Geometry check sheet. Reference: drawing and pictorial views, mm from the part's lowest x, y, z. A direction names the side the tool comes from. Give positions to 0.01 mm unless a question says otherwise; leave off trailing zeros. Write each loop counter-clockwise with the first axis right and the second up, starting at its lowest first coordinate (ties: lowest second). Pieces come first, ordered by that corner, then holes. Notation, with made-up numbers: (64, 60.25) -> (118, 60.25) arc R32 cw to (118, 93.25) -> close; hole circle Ø2 at (85, 55.5). An arc over 180 degrees is marked (long way). Answer as CSV lines item,"result".
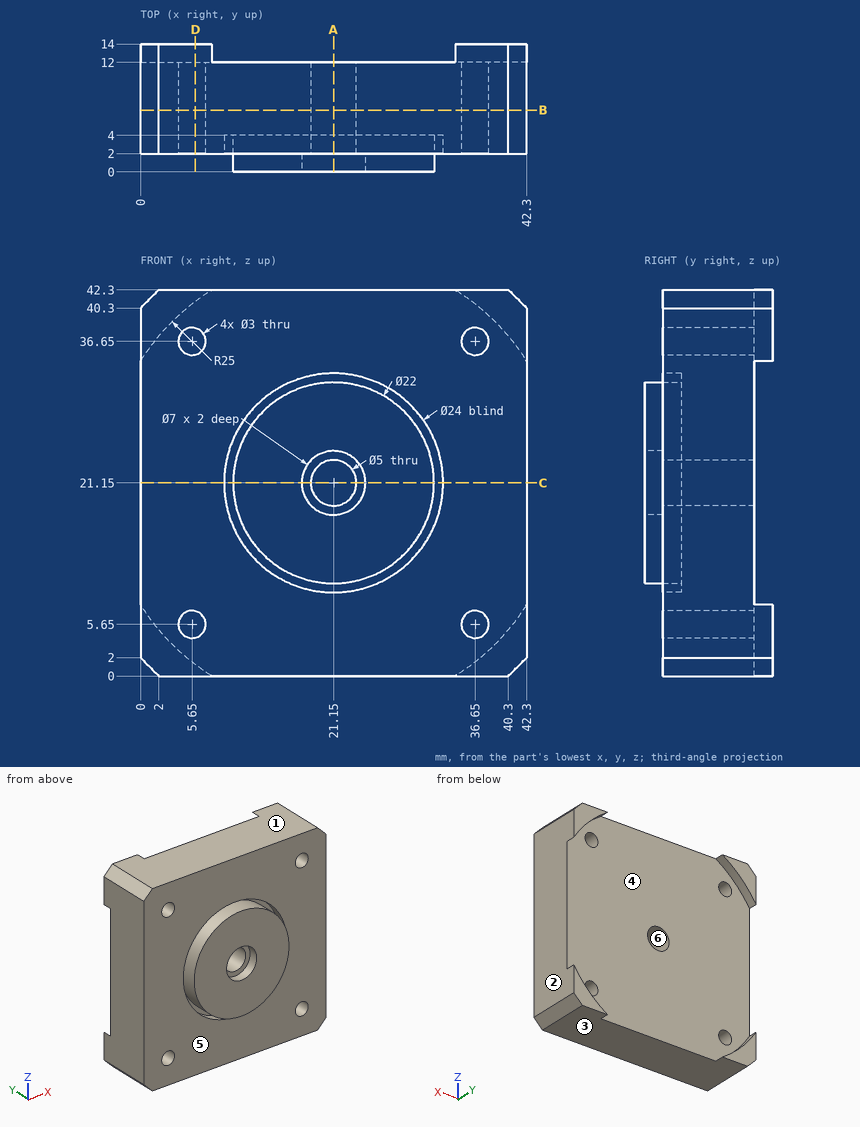
1) Section check B-B (y = 6.75). Record the boundary of the cut face in (x, z).
Reported:
outline,"(0, 2) -> (2, 0) -> (40.3, 0) -> (42.3, 2) -> (42.3, 40.3) -> (40.3, 42.3) -> (2, 42.3) -> (0, 40.3) -> close; hole circle Ø3 at (5.65, 5.65); hole circle Ø3 at (5.65, 36.65); hole circle Ø5 at (21.15, 21.15); hole circle Ø3 at (36.65, 5.65); hole circle Ø3 at (36.65, 36.65)"
2) Depth check by flat-ended pin: pin 1 (2 mm diameter, centred on x = 34, z = 5, fed in from +Y); pin 2 (5 mm diameter, centred on x = 5.65, z = 5.65, fed in from -Y). Enter the tip coordinate at first touch or a pass-through.
Reported:
pin 1,"y = 12"
pin 2,"y = 2"
3) Section check A-A (x = 21.15). Record the boundary of the cut face in (y, z).
Reported:
outline,"(0, 10.15) -> (4, 10.15) -> (4, 9.15) -> (2, 9.15) -> (2, 0) -> (12, 0) -> (12, 18.65) -> (2, 18.65) -> (2, 17.65) -> (0, 17.65) -> close; (0, 24.65) -> (2, 24.65) -> (2, 23.65) -> (12, 23.65) -> (12, 42.3) -> (2, 42.3) -> (2, 33.15) -> (4, 33.15) -> (4, 32.15) -> (0, 32.15) -> close"
4) Scan lines: line 1 along Z through (x, y) = (36.65, 5.25); line 2 along Z through (x, y) = (21.15, 6.75); line 3 along Z through (x, y) = (31, 3.75). Record each from-to range of solid material in increasing order.
Reported:
line 1,"0 to 4.15, 7.15 to 35.15, 38.15 to 42.3"
line 2,"0 to 18.65, 23.65 to 42.3"
line 3,"0 to 14.3, 16.25 to 26.05, 28 to 42.3"
5) Section check C-C (z = 21.15). Record the boundary of the cut face in (x, y).
Reported:
outline,"(0, 2) -> (9.15, 2) -> (9.15, 4) -> (10.15, 4) -> (10.15, 0) -> (17.65, 0) -> (17.65, 2) -> (18.65, 2) -> (18.65, 12) -> (0, 12) -> close; (23.65, 2) -> (24.65, 2) -> (24.65, 0) -> (32.15, 0) -> (32.15, 4) -> (33.15, 4) -> (33.15, 2) -> (42.3, 2) -> (42.3, 12) -> (23.65, 12) -> close"
6) Tool access check on the marked faces 5 and 6. Record the directions out of +Z, -Z, +X, -X, +Y, -Y that give a thin tool (end or side, any length) a straight path to the whole face; none if there is none.
Reported:
face 5,"-Y"
face 6,"+Y, -Y"
7) Draft check along Z on the marked faces 1, 2, 3 and 4. Enter one of: +Z half, -Z half, draft (parallel to the pull), parting line (faces both ways), or undercut.
Reported:
face 1,"+Z half"
face 2,"draft"
face 3,"-Z half"
face 4,"undercut"
8) Section check D-D (x = 6). Record the boundary of the cut face in (y, z).
Reported:
outline,"(2, 0) -> (14, 0) -> (14, 1.26) -> (12, 1.26) -> (12, 4.19) -> (2, 4.19) -> close; (2, 7.11) -> (12, 7.11) -> (12, 35.19) -> (2, 35.19) -> close; (2, 38.11) -> (12, 38.11) -> (12, 41.04) -> (14, 41.04) -> (14, 42.3) -> (2, 42.3) -> close"
